Part model, mm, in its own coordinate system. Face numbers are marked on the shaded views. A direction names the side the tool comes from. Round coordinates to 2 decimals unless told otherwise and drop trailing zeros. Loops run counter-clockwise (first coordinate to the right, second up) from the corner with the lowest first, then second, coordinate; pieces in that order, holes last. Notation, with made-up numbers: (32.25, 30.25) -> (46.25, 30.25) arc R34 cw to (46.25, 65.25) -> close; hole circle Ø6 at (8.5, 47). An arc over 180 degrees is marked (long way). Use a Markdown table: item, result. Add a question column.
Item 1: Flat gauge pins, fed straight in: pin 1 (1.6 mm diameter, centred on y = 1, z = 11, fed in from -X); pin 2 (1 mm diameter, centred on x = 29.5, z = 9, fed in from +Y); pin 3 (18.5 mm diameter, centred on x = 17.5, y = 34, fed in from -Z). Where does each tip first touch, or does it go through?
Item 2: Cut at D-D, the plane x = 9.5. List the corners of the cut face in (y, z).
Item 3: Cut at A-A, the plane x = 24.25. List the corners of the cut face in (y, z).
Item 4: Which spindle directions (+Z, -Z, +X, -X, +Y, -Y) get a long thin tool onto all of the face, cutting with end or side? Do the marked faces 1 and 2. Say none if no direction does.
Item 5: Probe line 1 (X direction, y = 37.75, z = 20.4); line 2 (X direction, y = 37.75, z = 19.5); line 3 (Y direction, x = 5, z = 19.9). List the from-to ranges inside material, lowest first. Write a range as [from, to].
Item 6: Cut at B-B, the plane y = 37.75. List the corners of the cut face in (x, z).
Item 7: Cut at C-C, the plane y = 43. List the corners of the cut face in (x, z), plus the area to 3 significant figures.
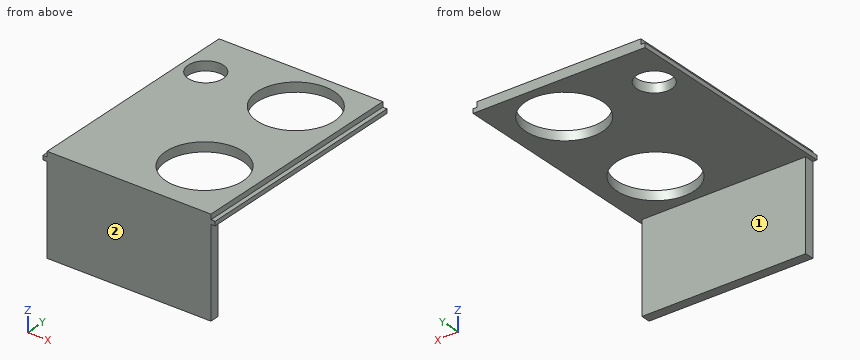
Autodesk Fusion 360 part; units mm, degrees
sketch "Sketch1" plane through (0, 0, 0) normal (0, 1, 0) x (1, 0, 0)
  line L0 (0, 0) -> (35, 0)
  line L1 (35, 0) -> (35, -19)
  line L2 (35, -19) -> (0, -19)
  line L3 (0, -19) -> (0, 0)
  line L4 (0, -19) -> (-0.9, -19)
  line L5 (-0.9, -19) -> (-0.9, -19.9)
  line L6 (-0.9, -19.9) -> (0, -19.9)
  line L7 (0, -19.9) -> (0, -21)
  line L8 (0, -21) -> (35, -21)
  line L9 (35, -21) -> (35, -19.9)
  line L10 (35, -19.9) -> (35.9, -19.9)
  line L11 (35.9, -19.9) -> (35.9, -19)
  line L12 (35.9, -19) -> (35, -19)
  dimension "d2" = 19
  dimension "d3" = 0.9
  dimension "d4" = 0.9
  dimension "d5" = 1.1
  dimension "d17" = 35
extrude "Extrude1" add sketch "Sketch1" along normal blind 48 contours L2 L4 L5 L6 L7 L8 L9 L10 L11 L12
extrude "Extrude2" add sketch "Sketch1" along normal blind 2 contours L0 L1 L2 L3
sketch "Sketch3" plane through (0, 0, 21) normal (0, 0, 1) x (-1, 0, 0)
  line L0 (0, 0) -> (-35, 0)
  line L1 (-35, 0) -> (-35, -48)
  line L2 (-35, -48) -> (0, -48)
  line L3 (0, -48) -> (0, 0)
  circle A0 centre (-24.25, -37.75) radius 8.25
  circle A1 centre (-24.25, -12.25) radius 8.25
  line L4 (-3, -46) -> (-36, -46) construction
  line L5 (-32.5, -48) -> (-32.5, 0) construction
  line L6 (-36, -4) -> (-3, -4) construction
  circle A2 centre (-5, -37.75) radius 3.75
  dimension "d10" = 16.5
  dimension "d11" = 2
  dimension "d12" = 2.5
  dimension "d13" = 42
  dimension "d14" = 7.5
  dimension "d15" = 5
extrude "Extrude3" cut sketch "Sketch3" against normal through all contours A0 | A1 | A2
A:
| question | item | result |
|---|---|---|
| 1 | pin 1 | stops at x = 0 |
| 1 | pin 2 | stops at y = 2 |
| 1 | pin 3 | stops at z = 19 |
| 2 | outline | (0, 0) -> (2, 0) -> (2, 19) -> (48, 19) -> (48, 21) -> (0, 21) -> close |
| 3 | outline | (0, 0) -> (2, 0) -> (2, 19) -> (4, 19) -> (4, 21) -> (0, 21) -> close; (20.5, 19) -> (29.5, 19) -> (29.5, 21) -> (20.5, 21) -> close; (46, 19) -> (48, 19) -> (48, 21) -> (46, 21) -> close |
| 4 | face 1 | -Z, +X, -X, +Y |
| 4 | face 2 | +Z, -Z, +X, -X, -Y |
| 5 | line 1 | x = [0, 1.25], [8.75, 16], [32.5, 35] |
| 5 | line 2 | x = [-0.9, 1.25], [8.75, 16], [32.5, 35.9] |
| 5 | line 3 | y = [0, 34], [41.5, 48] |
| 6 | outline | (-0.9, 19) -> (1.25, 19) -> (1.25, 21) -> (0, 21) -> (0, 19.9) -> (-0.9, 19.9) -> close; (8.75, 19) -> (16, 19) -> (16, 21) -> (8.75, 21) -> close; (32.5, 19) -> (35.9, 19) -> (35.9, 19.9) -> (35, 19.9) -> (35, 21) -> (32.5, 21) -> close |
| 7 | outline | (-0.9, 19) -> (17.89, 19) -> (17.89, 21) -> (0, 21) -> (0, 19.9) -> (-0.9, 19.9) -> close; (30.61, 19) -> (35.9, 19) -> (35.9, 19.9) -> (35, 19.9) -> (35, 21) -> (30.61, 21) -> close |
| 7 | area | 46.2 mm^2 |
